Autodesk Inventor part; units mm, degrees
ref_plane "YZ Plane" through (0, 0, 0) normal (1, 0, 0) x (0, 1, 0)
ref_plane "XZ Plane" through (0, 0, 0) normal (0, 1, 0) x (-1, 0, 0)
ref_plane "XY Plane" through (0, 0, 0) normal (0, 0, 1) x (1, 0, 0)
sketch "Sketch1" plane through (0, 0, 0) normal (0, 1, 0) x (-1, 0, 0)
  line L0 (0, 0) -> (85, 0)
  line L1 (85, 0) -> (85, -50)
  line L2 (85, -50) -> (0, -50)
  line L3 (0, -50) -> (0, 0)
  dimension "d0" = 85
  dimension "d1" = 50
extrude "Extrusion1" add sketch "Sketch1" along normal blind 25
sketch "Sketch2" plane through (0, 25, 0) normal (0, 1, 0) x (1, 0, 0)
  line L0 (-77.5, 26) -> (-7.5, 26)
  line L1 (-7.5, 26) -> (-7.5, 45)
  line L2 (-7.5, 45) -> (-77.5, 45)
  line L3 (-77.5, 45) -> (-77.5, 26)
  line L4 (-85, 50) -> (-85, 0)
  line L5 (0, 50) -> (-85, 50)
  point P0 (0, 0)
  dimension "d4" = 70
  dimension "d5" = 7.5
  dimension "d6" = 5
  dimension "d7" = 19
extrude "Extrusion2" cut sketch "Sketch2" against normal blind 20
fillet "Fillet1" radius 5 4 edges at (-85, 12.5, 0) (-85, 12.5, -50) (0, 12.5, -50) (0, 12.5, 0)
fillet "Fillet2" radius 7 2 edges at (-42.5, 5, -26) (-42.5, 5, -45)
properties part number "Web_server_holder"
Here's how the part is built. I have some questions about the finished solid (model axes, mm). A direction names the side the tool comes from. Round coordinates to 2 decimals unless told otherwise and drop trailing zeros. Loops run counter-clockwise (first coordinate to the right, second up) from the corner with the lowest first, then second, coordinate; pieces in that order, holes last. Notation, with made-up numbers: M 39,51 L 62,51 A10 ccw 62,58 Z; hole C 50,33.25 d3. An arc over 180 degrees is marked long. Write each question's results on one line, items separated by ' | '. Start each with the question number.
(1) Will these pins go through, and if not, where does the flat tip stop? P1, Ø10, axis at x = -41.5, z = -44, coming from the +Y side; P2, Ø1.5, axis at x = -58.5, z = -36, coming from the +Y side.
(2) Thinking about a two-plate mould opening in Z: for faces 1 (the flat face through (-42, 12, 0)), 2 (the cylindrical face through (-43, 7.1, -43)), 3 (the cylindrical face through (-83, 13, -49)), which applies, pulls with the +Z half, pulls with the -Z half, needs draft (parallel to the pull), parting line crosses it, or undercut?
(3) I want a section at A-A (y = 16). Please give me the cut outline in (x, z).
(4) I want a section at B-B (z = -36). Please give me the cut outline in (x, y).
(5) On a 3-axis mill with a long thin cutter (end or side, diameter ignored), from which of +Z, -Z, +X, -X, +Y, -Y can I reach the whole of each face in a straight line? I mean faces 4 (the flat face through (-42, 25, -19)), 5 (the flat face through (-43, 5, -36)). Say none if no direction works.
(6) I want a section at C-C (x = -22). Please give me the cut outline in (y, z), then the cut area to 3 significant figures.
(7) I want a section at D-D (y = 8). Please give me the cut outline in (x, z), then the cut area to 3 significant figures.
(8) If I drill on probe 1 along Z at (x, y) = (-11.5, 22.25); probe 2 along Z at (x, y) = (-55, 8); probe 3 along X at (y, z) = (11.5, -34), over which ranges is the centre line in solid material (lowest first)? Write a range as from..to.
Solved:
1) P1: stops at y = 25 | P2: stops at y = 5
2) face 1: pulls with the +Z half | face 2: undercut | face 3: pulls with the -Z half
3) outline: M -85,-45 A5 ccw -80,-50 L -5,-50 A5 ccw 0,-45 L 0,-5 A5 ccw -5,0 L -80,0 A5 ccw -85,-5 Z; hole M -77.5,-45 L -7.5,-45 L -7.5,-26 L -77.5,-26 Z
4) outline: M -85,0 L 0,0 L 0,25 L -7.5,25 L -7.5,5 L -77.5,5 L -77.5,25 L -85,25 Z
5) face 4: +Z, -Z, +X, -X, +Y | face 5: +Y
6) outline: M 0,-50 L 25,-50 L 25,-45 L 12,-45 A7 cw 5,-38 L 5,-33 A7 cw 12,-26 L 25,-26 L 25,0 L 0,0 Z | area: 891 mm²
7) outline: M -85,-45 A5 ccw -80,-50 L -5,-50 A5 ccw 0,-45 L 0,-5 A5 ccw -5,0 L -80,0 A5 ccw -85,-5 Z; hole M -77.5,-43.74 L -7.5,-43.74 L -7.5,-27.26 L -77.5,-27.26 Z | area: 3,070 mm²
8) probe 1: z = -50..-45, -26..0 | probe 2: z = -50..-43.74, -27.26..0 | probe 3: x = -85..-77.5, -7.5..0
